The listing builds one solid part. Answer for the finished solid, in the listing's coordinates (mm). A direction names the side the tool comes from. Coordinates: 2 decimals unless noted, no trailing zeros. Order: outer loops, then holes, each group sorted by start corner. A loop starts at its lowest first (then second) coordinate and runs counter-clockwise, first axis right, second up. Notation, with made-up numbers: M 83.5,-38 L 134.5,-38 A32 ccw 134.5,-4 Z; hole C 39,70 d4. An arc over 180 degrees is marked long. One line per item, written item: value. Start each with the question number.
Q1. The part is cut by section A-A on z = -3. Give the vertices of the cut face in (x, y), then the cut area to 3 significant figures.
Q2. The part is cut by section D-D on y = -18.5. Give the vertices of the cut face in (x, z).
Q3. Determine the mould class of faces 1 (the flat face through (-17.773, -38, 0)), 2 (the flat face through (0, -39.079, 0)), 3 (the flat face through (0, -36.079, -1)), 4 (the cylindrical face through (-0.67, -36.819, -1.383)) for opening direction X: pulls with the +X half, pulls with the -X half, needs draft (parallel to the pull), parting line crosses it, or undercut.
Q4. The part is cut by section B-B on x = 5. Give the vertices of the cut face in (y, z), then the cut area to 3 significant figures.
Q5. Straight lines are drawn through the part: line 1 along X through (y, z) = (-36.45, 0); line 2 along X through (y, z) = (-38.5, -3); line 3 along Y through (x, z) = (10.5, -4.25). For each, find the intervals that lie inside material, in ascending order. Write a range as [from, to].
Q6. Each of these flat-tipped pins is pushed along its axis until it touches: pin 1 Ø1.2 at (x, z) = (0, -3) entering from +Y; pin 2 Ø1 at (x, z) = (-11, -4) entering from +Y; pin 3 Ø3 at (x, z) = (-15.27, 0) entering from +Y; pin 4 Ø6 at (x, z) = (-4.5, -2) entering from +Y. Where does it stop, or does it pass through?
Q7. The part is cut by section C-C on z = 2.25. Give the vertices of the cut face in (x, y), then the cut area to 3 significant figures.
Q8. For faces 5 (the flat face through (-3.327, -24.007, 2.958)), 6 (the flat face through (3, -21, 0)), 7 (the flat face through (14, -37.579, 0)), determine the directions among +Z, -Z, +X, -X, +Y, -Y from which every point of the face is accessible in a straight line to the end or side of a thin tool.
```python
from build123d import *

# Parameters (mm, degrees)
EXTRUDE_1_DEPTH     = 6
SKETCH_3_W          = 35.546514436
SKETCH_3_H          = 12
EXTRUDE_2_DEPTH     = 3
SKETCH_1_5_R        = 1.2
CUT_EXTRUDE_1_DEPTH = 44.348392083
SKETCH_4_R          = 1.75
SKETCH_4_R_2        = 1
CUT_EXTRUDE_2_DEPTH = 1.5
SKETCH_4_2_R        = 1
CUT_EXTRUDE_3_DEPTH = 44.348392083


with BuildPart() as part:
    # Sketch 1 → Extrude 1 (new body)
    with BuildSketch(Plane.XY):
        with BuildLine():
            Line((0, -11.591109915), (6.561600135, -36.079335))
            Line((6.561600135, -36.079335), (12.773257218, -36.079335))
            Line((12.773257218, -36.079335), (2.897777479, 0.776457135))
            ThreePointArc((2.897777479, 0.776457135), (0, 3), (-2.897777479, 0.776457135))
            Line((-2.897777479, 0.776457135), (-12.773257218, -36.079335))
            Line((-12.773257218, -36.079335), (-6.561600135, -36.079335))
            Line((-6.561600135, -36.079335), (0, -11.591109915))
        make_face()
    extrude(amount=EXTRUDE_1_DEPTH)

    # Sketch 3 → Extrude 2 (add)
    with BuildSketch(Plane.XZ.offset(36.079335)):
        Rectangle(SKETCH_3_W, SKETCH_3_H)
    extrude(amount=EXTRUDE_2_DEPTH)

    # Sketch 1_5 → Cut-Extrude 1 (cut, through all)
    with BuildSketch(Plane.XY):
        Circle(SKETCH_1_5_R)
    extrude(amount=CUT_EXTRUDE_1_DEPTH, mode=Mode.SUBTRACT)

    # Sketch 4 → Cut-Extrude 2 (cut)
    # profile 1 of 3: a face of its own
    with BuildSketch(Plane(origin=(0, -36.079335, 0), x_dir=(1, 0, 0), z_dir=(0, 1, 0))):
        with Locations(Location((15.273257218, 0, 0), (0, 0, 270))):
            Circle(SKETCH_4_R)
        with Locations(Location((15.273257218, 0, 0), (0, 0, 270))):
            Circle(SKETCH_4_R_2, mode=Mode.SUBTRACT)
    # profile 2 of 3: a face of its own
    with BuildSketch(Plane(origin=(0, -36.079335, 0), x_dir=(1, 0, 0), z_dir=(0, 1, 0))):
        with Locations(Location((-15.273257218, 0, 0), (0, 0, 270))):
            Circle(SKETCH_4_R)
        with Locations(Location((-15.273257218, 0, 0), (0, 0, 270))):
            Circle(SKETCH_4_R_2, mode=Mode.SUBTRACT)
    # profile 3 of 3: a face of its own
    with BuildSketch(Plane(origin=(0, -36.079335, 0), x_dir=(1, 0, 0), z_dir=(0, 1, 0))):
        with Locations(Location((0, 3, 0), (0, 0, 270))):
            Circle(SKETCH_4_R)
        with Locations(Location((0, 3, 0), (0, 0, 270))):
            Circle(SKETCH_4_R_2, mode=Mode.SUBTRACT)
    extrude(amount=-CUT_EXTRUDE_2_DEPTH, mode=Mode.SUBTRACT)

    # Sketch 4_2 → Cut-Extrude 3 (cut, through all)
    with BuildSketch(Plane(origin=(0, -36.079335, 0), x_dir=(1, 0, 0), z_dir=(0, 1, 0))):
        with Locations(Location((15.273257218, 0, 0), (0, 0, 270))):
            Circle(SKETCH_4_2_R)
        with Locations(Location((0, 3, 0), (0, 0, 270))):
            Circle(SKETCH_4_2_R)
        with Locations(Location((-15.273257218, 0, 0), (0, 0, 270))):
            Circle(SKETCH_4_2_R)
    extrude(amount=-CUT_EXTRUDE_3_DEPTH, mode=Mode.SUBTRACT)


solid = part.part
```
Output:
1. outline: M -17.77,-39.08 L -1,-39.08 L -1,-37.58 L -1.75,-37.58 L -1.75,-36.08 L -17.77,-36.08 Z; M 1,-39.08 L 17.77,-39.08 L 17.77,-36.08 L 1.75,-36.08 L 1.75,-37.58 L 1,-37.58 Z
1. area: 98.4 mm^2
2. outline: M -8.06,0 L -1.85,0 L -1.85,6 L -8.06,6 Z; M 1.85,0 L 8.06,0 L 8.06,6 L 1.85,6 Z
3. face 1: pulls with the -X half
3. face 2: needs draft
3. face 3: undercut
3. face 4: undercut
4. outline: M -39.08,-6 L -36.08,-6 L -36.08,6 L -39.08,6 Z; M -30.25,0 L -7.07,0 L -7.07,6 L -30.25,6 Z
4. area: 175 mm^2
5. line 1: x = [-17.77, -17.02], [-13.52, 13.52], [17.02, 17.77]
5. line 2: x = [-17.77, -1], [1, 17.77]
5. line 3: y = [-39.08, -36.08]
6. pin 1: passes through
6. pin 2: stops at y = -36.08
6. pin 3: stops at y = -37.58
6. pin 4: stops at y = 1.97
7. outline: M -17.77,-39.08 L 17.77,-39.08 L 17.77,-36.08 L 12.77,-36.08 L 2.9,0.78 A3 ccw -2.9,0.78 L -12.77,-36.08 L -17.77,-36.08 Z; hole M -6.56,-36.08 L 6.56,-36.08 L 0,-11.59 Z; hole C 0,0 d2.4
7. area: 529 mm^2
8. face 5: +Z, -Z
8. face 6: -Z, +X, -X, +Y
8. face 7: +Y
